Geometry check sheet. Reference: the model listing, model coordinates, mm. A direction names the side the tool comes from. Give positions to 0.01 mm unless a question says otherwise; leave off trailing zeros. Order: outer loops, then holes, each group sorted by start corner. A loop starts at its lowest first (then second) coordinate and runs counter-clockwise, first axis right, second up. Notation, with made-up numbers: M 26,-38.5 L 80,-38.5 A22 ccw 80,-24.5 Z; hole C 74,-15.75 d1. An arc over 180 degrees is marked long. Answer as CSV lines item,"result". Start each with the question number.
```python
from build123d import *

# Parameters (mm, degrees)
SZKIC1_R                    = 6
DODANIE_WYCI_GNI_CIE1_DEPTH = 3
SZKIC4_R                    = 9.75
SZKIC4_R_2                  = 6.5
DODANIE_WYCI_GNI_CIE2_DEPTH = 2.5


with BuildPart() as part:
    # Szkic1 → Dodanie-wyciągnięcie1 (new, symmetric)
    with BuildSketch(Plane(origin=(0, 0, 0), x_dir=(1, 0, 0), z_dir=(0, 1, 0))):
        Polygon((9.5, -5.484827557), (9.5, 5.484827557), (0, 10.969655115), (-9.5, 5.484827557), (-9.5, -5.484827557), (0, -10.969655115), align=None)
        with Locations(Location((0, 0, 0), (0, 0, 270))):
            Circle(SZKIC1_R, mode=Mode.SUBTRACT)
    extrude(amount=DODANIE_WYCI_GNI_CIE1_DEPTH, both=True)

    # Szkic3 → Wycięcie-obrót9 (revolve, cut)
    with BuildSketch(Plane(origin=(0, 0, 0), x_dir=(0, 0, -1), z_dir=(1, 0, 0))):
        Polygon((10.969655115, 3), (10.969655115, 2), (9.969655115, 3), align=None)
        Polygon((9.969655115, -3), (10.969655115, -3), (10.969655115, -2), align=None)
    revolve(axis=Axis((0, 0, 0), (0, 1, 0)), mode=Mode.SUBTRACT)

    # Szkic4 → Dodanie-wyciągnięcie2 (add)
    with BuildSketch(Plane(origin=(0, 3, 0), x_dir=(1, 0, 0), z_dir=(0, 1, 0))):
        with Locations(Location((0, 0, 0), (0, 0, 106.997175533))):
            Circle(SZKIC4_R)
        with Locations(Location((0, 0, 0), (0, 0, 270))):
            Circle(SZKIC4_R_2, mode=Mode.SUBTRACT)
    extrude(amount=DODANIE_WYCI_GNI_CIE2_DEPTH)


solid = part.part
```
Item 1: Section check D-D on y = 4.25. Record the boundary of the cut face in (x, z).
Item 2: Section check A-A on z = 0. Record the boundary of the cut face in (x, y), then the cut area to 4 significant figures.
Item 3: Section check B-B on y = -1. Record the boundary of the cut face in (x, z).
Item 4: Section check C-C on x = 3.5. Record the boundary of the cut face in (y, z).
Item 5: Scan lines: line 1 along X through (y, z) = (0.4, 0); line 2 along X through (y, z) = (3.6, 0); line 3 along Z through (x, y) = (5, 1). Record each from-to range of solid material in increasing order.
Item 6: Depth check by flat-ended pin: pin 1 Ø8 at (x, z) = (0, 0) entering from +Y; pin 2 Ø1.8 at (y, z) = (-1.5, -1) entering from -X; pin 3 Ø2 at (x, y) = (7, -1.5) entering from -Z. Enter the tip coordinate at first touch or a pass-through.
Item 7: Access from +Z, -Z, +X, -X, +Y, -Y to the whole of each face (thin tool, end or side, straight path). Record for faces 1 (the face through (4.684, 0.042, 8.266)), 2 (the face through (-4, -3, -5)).
Item 8: Draft check along Z on faces 3 (the face through (-4.684, 0.042, -8.266)), 4 (the face through (-0.03, -2.73, 10.24)), 5 (the face through (7.935, 4.232, 5.665)), 6 (the face through (-3.955, 4.232, -5.158)). Enter one of: pulls with the +Z half, pulls with the -Z half, needs draft (parallel to the pull), parting line crosses it, or undercut.
Numbers:
1,outline,"C 0,0 d19.5; hole C 0,0 d13"
2,outline,"M -9.75,3 L -9.5,3 L -9.5,-3 L -6,-3 L -6,3 L -6.5,3 L -6.5,5.5 L -9.75,5.5 Z; M 6,-3 L 9.5,-3 L 9.5,3 L 9.75,3 L 9.75,5.5 L 6.5,5.5 L 6.5,3 L 6,3 Z"
2,area,"58.25 mm2"
3,outline,"M -9.5,-5.48 L 0,-10.97 L 9.5,-5.48 L 9.5,5.48 L 0,10.97 L -9.5,5.48 Z; hole C 0,0 d12"
4,outline,"M -3,-8.95 L 3,-8.95 L 3,-9.1 L 5.5,-9.1 L 5.5,-5.48 L 3,-5.48 L 3,-4.87 L -3,-4.87 Z; M -3,4.87 L 3,4.87 L 3,5.48 L 5.5,5.48 L 5.5,9.1 L 3,9.1 L 3,8.95 L -3,8.95 Z"
5,line 1,"-9.5 to -6, 6 to 9.5"
5,line 2,"-9.75 to -6.5, 6.5 to 9.75"
5,line 3,"-8.08 to -3.32, 3.32 to 8.08"
6,pin 1,"through"
6,pin 2,"x = -9.5"
6,pin 3,"z = -7.51"
7,face 1,"+Z, +X, -Y"
7,face 2,"+Z, -Z, +X, -X, -Y"
8,face 3,"pulls with the -Z half"
8,face 4,"pulls with the +Z half"
8,face 5,"parting line crosses it"
8,face 6,"undercut"
